```python
from build123d import *

# Parameters (mm, degrees)
SKETCH1_R            = 11.825
MAIN_STRUCTURE_DEPTH = 50
SKETCH2_R            = 8.825
HOLE_DEPTH           = 15.5
STRUCTURE_FILLET_R   = 1
CUT_EXTRUDE1_REACH   = 54.722
SKETCH3_R            = 0.795


with BuildPart() as part:
    # Sketch1 → Main Structure (new body)
    with BuildSketch(Plane(origin=(0, 0, 0), x_dir=(1, 0, 0), z_dir=(0, 1, 0))):
        with Locations(Location((0, 0, 0), (0, 0, 270))):
            Circle(SKETCH1_R)
    extrude(amount=MAIN_STRUCTURE_DEPTH)

    # Sketch2 → Hole (cut)
    with BuildSketch(Plane(origin=(0, 50, 0), x_dir=(1, 0, 0), z_dir=(0, 1, 0))):
        with Locations(Location((0, 0, 0), (0, 0, 270))):
            Circle(SKETCH2_R)
    extrude(amount=-HOLE_DEPTH, mode=Mode.SUBTRACT)

    # Structure Fillet
    structure_fillet_edges = [part.edges().sort_by_distance(p)[0] for p in [
        (0, 50, -11.825),
    ]]
    fillet(structure_fillet_edges, radius=STRUCTURE_FILLET_R)

    # Sketch3 → Cut-Extrude1 (cut, up to next)
    with BuildSketch(Plane.XZ, mode=Mode.PRIVATE) as cut_extrude1_sk1:
        with Locations(Location((0, 0, 0), (0, 0, 270))):
            Circle(SKETCH3_R)
    cut_extrude1_tool1 = extrude(cut_extrude1_sk1.sketch, amount=-CUT_EXTRUDE1_REACH, mode=Mode.PRIVATE) & part.part
    add(cut_extrude1_tool1.solids().sort_by_distance((0, 0, 0))[0], mode=Mode.SUBTRACT)


solid = part.part
```
Here's how the part is built. I have some questions about the finished solid (model axes, mm). A direction names the side the tool comes from. Coordinates: 2 decimals unless noted, no trailing zeros. Order: outer loops, then holes, each group sorted by start corner. A loop starts at its lowest first (then second) coordinate and runs counter-clockwise, first axis right, second up.
Item 1: Which directions (+Z, -Z, +X, -X, +Y, -Y) give clear straight access to the entire face, cutting with the end or side of a thin tool? Please do faces 1 (the face through (-2, 0, 0)), 2 (the face through (-2, 34.5, 0)).
Response values:
face 1: +Z, -Z, +X, -X, -Y
face 2: +Y
Item 2: If we section it at B-B, the plane x = 0: List the corners of the cut face in (y, z) for me (3 decimals), then the cut area to 3 significant figures.
Response values:
outline: (0, -11.825) - (49, -11.825) arc R1 ccw to (50, -10.825) - (50, -8.825) - (34.5, -8.825) - (34.5, -0.795) - (0, -0.795) - close; (0, 0.795) - (34.5, 0.795) - (34.5, 8.825) - (50, 8.825) - (50, 10.825) arc R1 ccw to (49, 11.825) - (0, 11.825) - close
area: 854 mm2
Item 3: If we section it at C-C, the plane y = 20.5: List the corners of the cut face in (x, z) for me (3 decimals).
Response values:
outline: circle Ø23.65 at (0, 0); hole circle Ø1.59 at (0, 0)
Item 4: I'm going to push flat-ended pins straight in: pin 1 Ø2 at (x, y) = (-9, 30) entering from +Z; pin 2 Ø5.5 at (x, z) = (3.5, -3.5) entering from +Y; pin 3 Ø1.5 at (x, y) = (-4.5, 26.5) entering from -Z. Where does each tip first touch, or does it pass through?
Response values:
pin 1: stops at z = 8.71
pin 2: stops at y = 34.5
pin 3: stops at z = -11.21
Item 5: Thinking about a two-plate mould opening in X: for faces 3 (the face through (-11.544, 24.157, -2.563)), 4 (the face through (-0.776, 17.008, 0.172)), 5 (the face through (0, 50, -9)), which applies, pulls with the +X half, pulls with the -X half, needs draft (parallel to the pull), parting line crosses it, or undercut?
Response values:
face 3: parting line crosses it
face 4: undercut
face 5: needs draft
Item 6: I need wall thicknesses on probe 1 along X at (y, z) = (24.5, 0) (3 decimals); probe 2 along X at (y, z) = (45, 0) (3 decimals); probe 3 along Y at (x, z) = (-4.25, -6.5). Which ranges of each line are inside material? Lowest first, please.
Response values:
probe 1: x = -11.825 to -0.795, 0.795 to 11.825
probe 2: x = -11.825 to -8.825, 8.825 to 11.825
probe 3: y = 0 to 34.5
Item 7: If we section it at A-A, the plane z = 0: List the corners of the cut face in (x, y) for me (3 decimals), then the cut area to 3 significant figures.
Response values:
outline: (-11.825, 0) - (-0.795, 0) - (-0.795, 34.5) - (-8.825, 34.5) - (-8.825, 50) - (-10.825, 50) arc R1 ccw to (-11.825, 49) - close; (0.795, 0) - (11.825, 0) - (11.825, 49) arc R1 ccw to (10.825, 50) - (8.825, 50) - (8.825, 34.5) - (0.795, 34.5) - close
area: 854 mm2
